from build123d import *

# Parameters (mm, degrees)
EXTRUSION1_DEPTH       = 2.5
EXTRUSION1_DEPTH_BACK  = 2.5
SKETCH1_R              = 172.5
EXTRUSION2_DEPTH       = 244.964649079
EXTRUSION2_DEPTH_BACK  = 244.964649079
EXTRUSION3_DEPTH       = 240.778543661
EXTRUSION3_DEPTH_BACK  = 240.778543661
EXTRUSION4_DEPTH       = 239.196347579
EXTRUSION4_DEPTH_BACK  = 239.196347579
EXTRUSION8_DEPTH       = 239.196347579
EXTRUSION8_DEPTH_BACK  = 239.196347579
SKETCH7_R              = 2.5
EXTRUSION9_DEPTH       = 239.196347579
EXTRUSION9_DEPTH_BACK  = 239.196347579
SKETCH8_R              = 2.5
EXTRUSION10_DEPTH      = 239.196347579
EXTRUSION10_DEPTH_BACK = 239.196347579
SKETCH9_R              = 2.5
EXTRUSION11_DEPTH      = 5
SKETCH11_R             = 2.5
SKETCH11_R_2           = 2.51471315
CUT_EXTRUDE1_DEPTH     = 27


with BuildPart() as part:
    # Sketch1 → Extrusion1 (new, two sides: drawn at the far end of the back side and taken through both)
    with BuildSketch(Plane(origin=(0, 0, 0), x_dir=(-1, 0, 0), z_dir=(0, 1, 0)).offset(-EXTRUSION1_DEPTH_BACK)):
        with Locations(Location((0, 0, 0), (0, 0, 90))):
            Circle(SKETCH1_R)
    extrude(amount=EXTRUSION1_DEPTH + EXTRUSION1_DEPTH_BACK)

    # Sketch2 → Extrusion2 (cut, two sides: drawn at the far end of the back side and taken through both)
    with BuildSketch(Plane(origin=(0, 0, 0), x_dir=(1, 0, 0), z_dir=(0, 1, 0)).offset(-EXTRUSION2_DEPTH_BACK)):
        with BuildLine():
            Line((45, -166.527024834), (-45, -166.527024834))
            ThreePointArc((-45, -166.527024834), (0, -172.5), (45, -166.527024834))
        make_face()
        with BuildLine():
            Line((-45, 166.527024834), (45, 166.527024834))
            ThreePointArc((45, 166.527024834), (0, 172.5), (-45, 166.527024834))
        make_face()
        with BuildLine():
            Line((-170.293863659, -27.5), (-170.293863659, 27.5))
            ThreePointArc((-170.293863659, 27.5), (-172.5, 0), (-170.293863659, -27.5))
        make_face()
    extrude(amount=EXTRUSION2_DEPTH + EXTRUSION2_DEPTH_BACK, mode=Mode.SUBTRACT)

    # Sketch3 → Extrusion3 (cut, two sides: drawn at the far end of the back side and taken through both)
    with BuildSketch(Plane(origin=(0, 0, 0), x_dir=(1, 0, 0), z_dir=(0, 1, 0)).offset(-EXTRUSION3_DEPTH_BACK)):
        with BuildLine():
            Line((170.293863659, -27.5), (170.293863659, 27.5))
            ThreePointArc((170.293863659, 27.5), (172.5, 0), (170.293863659, -27.5))
        make_face()
    extrude(amount=EXTRUSION3_DEPTH + EXTRUSION3_DEPTH_BACK, mode=Mode.SUBTRACT)

    # Sketch4 → Extrusion4 (cut, two sides: drawn at the far end of the back side and taken through both)
    with BuildSketch(Plane(origin=(0, 0, 0), x_dir=(1, 0, 0), z_dir=(0, 1, 0)).offset(-EXTRUSION4_DEPTH_BACK)):
        with BuildLine():
            ThreePointArc((170.293863659, -27.5), (134.081167118, -56.402573756), (138.744369255, -102.5))
            ThreePointArc((138.744369255, -102.5), (159.00442557, -66.886789797), (170.293863659, -27.5))
        make_face()
        with BuildLine():
            ThreePointArc((170.293863659, 27.5), (159.00442557, 66.886789797), (138.744369255, 102.5))
            ThreePointArc((138.744369255, 102.5), (134.081167118, 56.402573756), (170.293863659, 27.5))
        make_face()
    extrude(amount=EXTRUSION4_DEPTH + EXTRUSION4_DEPTH_BACK, mode=Mode.SUBTRACT)

    # Sketch7 → Extrusion8 (cut, two sides: drawn at the far end of the back side and taken through both)
    with BuildSketch(Plane(origin=(0, 0, 0), x_dir=(1, 0, 0), z_dir=(0, 1, 0)).offset(-EXTRUSION8_DEPTH_BACK)):
        with Locations(Location((-162.793863659, -15, 0), (0, 0, 270))):
            Circle(SKETCH7_R)
        with Locations(Location((-162.793863659, 0, 0), (0, 0, 270))):
            Circle(SKETCH7_R)
        with Locations(Location((-162.793863659, 15, 0), (0, 0, 270))):
            Circle(SKETCH7_R)
    extrude(amount=EXTRUSION8_DEPTH + EXTRUSION8_DEPTH_BACK, mode=Mode.SUBTRACT)

    # Sketch8 → Extrusion9 (cut, two sides: drawn at the far end of the back side and taken through both)
    with BuildSketch(Plane(origin=(0, 0, 0), x_dir=(1, 0, 0), z_dir=(0, 1, 0)).offset(-EXTRUSION9_DEPTH_BACK)):
        with Locations(Location((-15, -159.027024834, 0), (0, 0, 270))):
            Circle(SKETCH8_R)
        with Locations(Location((0, -159.027024834, 0), (0, 0, 270))):
            Circle(SKETCH8_R)
        with Locations(Location((15, -159.027024834, 0), (0, 0, 270))):
            Circle(SKETCH8_R)
    extrude(amount=EXTRUSION9_DEPTH + EXTRUSION9_DEPTH_BACK, mode=Mode.SUBTRACT)

    # Sketch9 → Extrusion10 (cut, two sides: drawn at the far end of the back side and taken through both)
    with BuildSketch(Plane(origin=(0, 0, 0), x_dir=(1, 0, 0), z_dir=(0, 1, 0)).offset(-EXTRUSION10_DEPTH_BACK)):
        with Locations(Location((0.205214566, 159.027024834, 0), (0, 0, 270))):
            Circle(SKETCH9_R)
        with Locations(Location((-14.794785434, 159.027024834, 0), (0, 0, 270))):
            Circle(SKETCH9_R)
        with Locations(Location((15.205214566, 159.027024834, 0), (0, 0, 270))):
            Circle(SKETCH9_R)
    extrude(amount=EXTRUSION10_DEPTH + EXTRUSION10_DEPTH_BACK, mode=Mode.SUBTRACT)

    # Sketch10 → Extrusion11 (add)
    with BuildSketch(Plane(origin=(0, 0, 0), x_dir=(1, 0, 0), z_dir=(0, 1, 0))):
        with BuildLine():
            Line((120.84, -99.290756871), (120.84, 99.290756871))
            ThreePointArc((120.84, 99.290756871), (-156.4, 0), (120.84, -99.290756871))
        make_face()
        with BuildLine():
            ThreePointArc((116.84, 97.847710244), (-152.4, 0), (116.84, -97.847710244))
            Line((116.84, -97.847710244), (116.84, 97.847710244))
        make_face(mode=Mode.SUBTRACT)
    extrude(amount=EXTRUSION11_DEPTH)

    # Sketch11 → Cut-Extrude1 (cut)
    with BuildSketch(Plane(origin=(0, -2.5, 0), x_dir=(-1, 0, 0), z_dir=(0, -1, 0))):
        with Locations(Location((114.237315354, 61.453329839, 0), (0, 0, 90))):
            Circle(SKETCH11_R)
        with Locations(Location((114.237315354, 36.453329839, 0), (0, 0, 90))):
            Circle(SKETCH11_R)
        with Locations(Location((114.237315354, 11.453329839, 0), (0, 0, 90))):
            Circle(SKETCH11_R)
        with Locations(Location((114.237315354, -13.546670161, 0), (0, 0, 90))):
            Circle(SKETCH11_R)
        with Locations(Location((114.237315354, -38.546670161, 0), (0, 0, 90))):
            Circle(SKETCH11_R)
        with Locations(Location((83.382192066, 95.959187947, 0), (0, 0, 90))):
            Circle(SKETCH11_R)
        with Locations(Location((74.039046315, 112.7789931, 0), (0, 0, 90))):
            Circle(SKETCH11_R)
        with Locations(Location((59.896910692, 98.636857477, 0), (0, 0, 90))):
            Circle(SKETCH11_R)
        with Locations(Location((-10.262684646, 74.659187947, 0), (0, 0, 90))):
            Circle(SKETCH11_R)
        with Locations(Location((-10.262684646, -34.140812053, 0), (0, 0, 90))):
            Circle(SKETCH11_R)
        with Locations(Location((-10.262684646, -49.740812053, 0), (0, 0, 90))):
            Circle(SKETCH11_R)
        with Locations(Location((-77.94, -64.847710244, 0), (0, 0, 90))):
            Circle(SKETCH11_R)
        with Locations(Location((-77.94, -44.847710244, 0), (0, 0, 90))):
            Circle(SKETCH11_R)
        with Locations(Location((-77.94, -24.847710244, 0), (0, 0, 90))):
            Circle(SKETCH11_R_2)
        with Locations(Location((-77.94, -4.847710244, 0), (0, 0, 90))):
            Circle(SKETCH11_R)
        with Locations(Location((-77.94, 15.152289756, 0), (0, 0, 90))):
            Circle(SKETCH11_R)
        with Locations(Location((-77.94, 35.152289756, 0), (0, 0, 90))):
            Circle(SKETCH11_R)
        with Locations(Location((-86.382165944, 95.260023358, 0), (0, 0, 90))):
            Circle(SKETCH11_R)
        with Locations(Location((-68.256010203, 103.712388593, 0), (0, 0, 90))):
            Circle(SKETCH11_R)
        with Locations(Location((-50.129854462, 112.164753828, 0), (0, 0, 90))):
            Circle(SKETCH11_R)
        with Locations(Location((-32.003698722, 120.617119063, 0), (0, 0, 90))):
            Circle(SKETCH11_R)
        with Locations(Location((-13.877542981, 129.069484298, 0), (0, 0, 90))):
            Circle(SKETCH11_R)
        with Locations(Location((4.24861276, 137.521849532, 0), (0, 0, 90))):
            Circle(SKETCH11_R)
        with Locations(Location((14.693361821, -98.240812053, 0), (0, 0, 90))):
            Circle(SKETCH11_R)
        with Locations(Location((14.693361821, -116.240812053, 0), (0, 0, 90))):
            Circle(SKETCH11_R)
        with Locations(Location((-58.218731113, -116.240812053, 0), (0, 0, 90))):
            Circle(SKETCH11_R)
        with Locations(Location((-58.218731113, -98.240812053, 0), (0, 0, 90))):
            Circle(SKETCH11_R)
        with Locations(Location((-19.084661413, 39.809187947, 0), (0, 0, 90))):
            Circle(SKETCH11_R)
        with Locations(Location((-19.084661413, 6.409187947, 0), (0, 0, 90))):
            Circle(SKETCH11_R)
    extrude(amount=-CUT_EXTRUDE1_DEPTH, mode=Mode.SUBTRACT)


solid = part.part
Geometry check sheet. Reference: the model listing, model coordinates, mm. A direction names the side the tool comes from. Round coordinates to 2 decimals unless told otherwise and drop trailing zeros. Loops run counter-clockwise (first coordinate to the right, second up) from the corner with the lowest first, then second, coordinate; pieces in that order, holes last. Notation, with made-up numbers: (27.5, -9.5) - (85.5, -9.5) arc R20 cw to (85.5, 26.5) - close; hole circle Ø3 at (-34, 4). An arc over 180 degrees is marked (long way). One line per question, with ' | ' between items. Start each with the question number.
1. Scan lines: line 1 (X direction, y = -0.75, z = -17); line 2 (X direction, y = -0.75, z = -34.5); line 3 (Y direction, x = 66.5, z = -16.5). Record each from-to range of solid material in increasing order. Write a range as [from, to].
2. Depth check by flat-ended pin: pin 1 (4 mm diameter, centred on x = 25.5, z = -22.5, fed in from +Y); pin 2 (4 mm diameter, centred on y = 1, z = 69.5, fed in from +X); pin 3 (1.2 mm diameter, centred on y = 3.5, z = 43, fed in from +X). Enter the tip coordinate at first touch or a pass-through.
3. Draft check along Z on faces 1 (the face through (-152.31, 3.73, -5.21)), 2 (the face through (134.35, -0.03, 55.78)), 3 (the face through (96.62, -0.04, 142.9)), 4 (the face through (-127.209, -0.035, -116.508)). Enter one of: released by +Z, released by -Z, zero draft, split by the parting line, or undercut.
4. Cross-section at A-A on z = -23. Record the cut outline in (x, y).
5. Tool access check on faces 5 (the face through (-156.308, 3.732, -5.372)), 6 (the face through (97.958, -0.035, -141.988)). Record the directions out of +Z, -Z, +X, -X, +Y, -Y that give a thin tool (end or side, any length) a straight path to the whole face; none if there is none.
Taken from the geometry:
1) line 1: [-170.29, -164.29], [-161.29, 76.26], [79.62, 170.29] | line 2: [-169.01, -115.8], [-112.68, 75.53], [80.35, 152.45] | line 3: [-2.5, 2.5]
2) pin 1: y = 2.5 | pin 2: x = 130.91 | pin 3: x = 120.84
3) face 1: undercut | face 2: undercut | face 3: released by +Z | face 4: released by -Z
4) outline: (-170.29, -2.5) - (170.29, -2.5) - (170.29, 2.5) - (120.84, 2.5) - (120.84, 5) - (116.84, 5) - (116.84, 2.5) - (-150.65, 2.5) - (-150.65, 5) - (-154.7, 5) - (-154.7, 2.5) - (-170.29, 2.5) - close
5) face 5: +Y | face 6: -Z, +X, +Y, -Y
